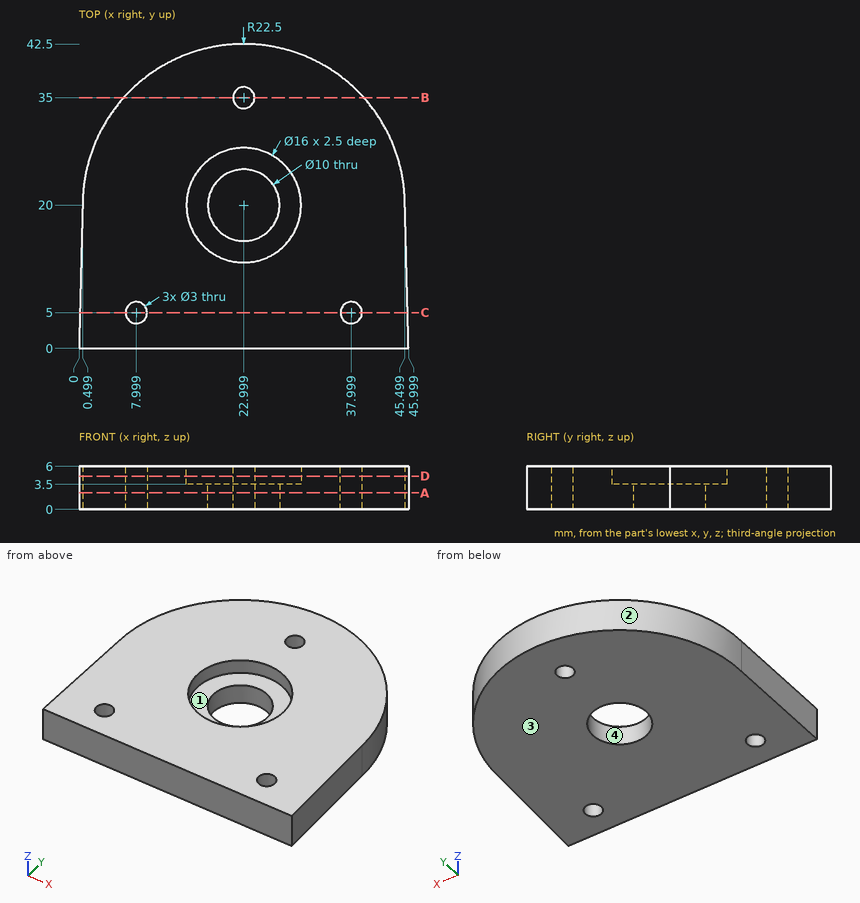
For this review, use the dimensioned drawing (mm, ordinates from the lowest corner) and the shaded views. Round coordinates to 2 decimals unless told otherwise and drop trailing zeros. Loops run counter-clockwise (first coordinate to the right, second up) from the corner with the lowest first, then second, coordinate; pieces in that order, holes last. Notation, with made-up numbers: (-34.5, -1.75) -> (-13.5, -1.75) arc R25 ccw to (-13.5, 16.25) -> close; hole circle Ø7 at (-13.5, -2). An arc over 180 degrees is marked (long way). Write item = value, one per line. Start each with the question number.
Item 1: Take a section at D-D on z = 4.65. Give the boundary of the cut face in (x, y), plus the area to 3 significant figures.
Item 2: To check wall thickness, follow L1, parallel to Z at x = 29.5, y = 22.5; L2, parallel to Y at x = 19, z = 1.5 (1 decimal); L3, parallel to Y at x = 38, z = 5.75. State the ranges of each line that lie inside material, in increasing order.
Item 3: Take a section at B-B on y = 35. Give the boundary of the cut face in (x, z).
Item 4: Insertion check: pin 1 (14.5 mm diameter, centred on x = 23, y = 20, fed in from +Z). The pin has a flat end and moves straight along its axis. Give the tip position at first contact, or say it passes through.
Item 5: Take a section at C-C on y = 5. Give the boundary of the cut face in (x, z) (1 decimal).
Item 6: Mouldability with a two-part tool opening along Y and no side actions: class the marked faces 1, 2, 3 and 4 as released by +Y, released by -Y, zero draft, split by the parting line, or undercut.
Item 7: Take a section at A-A on z = 2.3. Give the boundary of the cut face in (x, y), plus the area to 3 significant figures.
Result:
q1.outline = (0, 0) -> (46, 0) -> (45.5, 20) arc R22.5 ccw to (0.5, 20) -> close; hole circle Ø3 at (8, 5); hole circle Ø16 at (23, 20); hole circle Ø3 at (23, 35); hole circle Ø3 at (38, 5)
q1.area = 1,480 mm²
q2.L1 = 0 to 3.5
q2.L2 = 0 to 17, 23 to 42.1
q2.L3 = 0 to 3.5, 6.5 to 36.77
q3.outline = (6.23, 0) -> (21.5, 0) -> (21.5, 6) -> (6.23, 6) -> close; (24.5, 0) -> (39.77, 0) -> (39.77, 6) -> (24.5, 6) -> close
q4.pin_1 = 3.5
q5.outline = (0.1, 0) -> (6.5, 0) -> (6.5, 6) -> (0.1, 6) -> close; (9.5, 0) -> (36.5, 0) -> (36.5, 6) -> (9.5, 6) -> close; (39.5, 0) -> (45.9, 0) -> (45.9, 6) -> (39.5, 6) -> close
q6.face_1 = undercut
q6.face_2 = released by +Y
q6.face_3 = zero draft
q6.face_4 = undercut
q7.outline = (0, 0) -> (46, 0) -> (45.5, 20) arc R22.5 ccw to (0.5, 20) -> close; hole circle Ø3 at (8, 5); hole circle Ø10 at (23, 20); hole circle Ø3 at (23, 35); hole circle Ø3 at (38, 5)
q7.area = 1,610 mm²
